```python
from build123d import *

# Parameters (mm, degrees)
BOSS_EXTRUDE1_DEPTH = 1
SKETCH3_R           = 6.8
CUT_EXTRUDE1_DEPTH  = 10


with BuildPart() as part:
    # Sketch1 → Boss-Extrude1 (new body)
    with BuildSketch(Plane(origin=(0, 0, 0), x_dir=(1, 0, 0), z_dir=(0, 1, 0))):
        with BuildLine():
            Line((-58.095782979, 0), (-58.073036978, 0))
            ThreePointArc((-58.073036978, 0), (-57.597480623, -0.18634043), (-57.375111056, -0.646153846))
            ThreePointArc((-57.375111056, -0.646153846), (-48.676683494, -8.393775458), (-40.6, 0))
            Line((-40.6, 0), (-26.532998323, 0))
            ThreePointArc((-26.532998323, 0), (-23.34157463, 1.150998205), (-21.619480115, 4.074074074))
            ThreePointArc((-21.619480115, 4.074074074), (-7.819670385, 20.563383843), (13.44973545, 17.409899952))
            ThreePointArc((13.44973545, 17.409899952), (19.920363156, 17.713546888), (20.660984848, 24.148817192))
            ThreePointArc((20.660984848, 24.148817192), (-17.408618139, 43.353494129), (-53.539393939, 20.711026772))
            ThreePointArc((-53.539393939, 20.711026772), (-54.448939175, 20.409991078), (-54.807009858, 21.298630718))
            ThreePointArc((-54.807009858, 21.298630718), (-6.094732075, 58.483281722), (49.237842792, 32.141481565))
            ThreePointArc((49.237842792, 32.141481565), (49.203069762, 31.327605826), (48.421551499, 31.097753513))
            ThreePointArc((48.421551499, 31.097753513), (38.168934267, 19.364205559), (53.692695632, 20.707760837))
            ThreePointArc((53.692695632, 20.707760837), (54.339746442, 21.20266298), (55.017049011, 20.750043811))
            ThreePointArc((55.017049011, 20.750043811), (57.781950674, 10.894318531), (58.795732172, 0.708433735))
            ThreePointArc((58.795732172, 0.708433735), (58.593730574, 0.208016065), (58.095782979, 0))
            Line((58.095782979, 0), (58.073036978, 0))
            ThreePointArc((58.073036978, 0), (57.597480623, 0.18634043), (57.375111056, 0.646153846))
            ThreePointArc((57.375111056, 0.646153846), (48.676683494, 8.393775458), (40.6, 0))
            Line((40.6, 0), (26.532998323, 0))
            ThreePointArc((26.532998323, 0), (23.34157463, -1.150998205), (21.619480115, -4.074074074))
            ThreePointArc((21.619480115, -4.074074074), (7.819670385, -20.563383843), (-13.44973545, -17.409899952))
            ThreePointArc((-13.44973545, -17.409899952), (-19.920363156, -17.713546888), (-20.660984848, -24.148817192))
            ThreePointArc((-20.660984848, -24.148817192), (17.408618139, -43.353494129), (53.539393939, -20.711026772))
            ThreePointArc((53.539393939, -20.711026772), (54.448939175, -20.409991078), (54.807009858, -21.298630718))
            ThreePointArc((54.807009858, -21.298630718), (6.094732075, -58.483281722), (-49.237842792, -32.141481565))
            ThreePointArc((-49.237842792, -32.141481565), (-49.203069762, -31.327605826), (-48.421551499, -31.097753513))
            ThreePointArc((-48.421551499, -31.097753513), (-38.168934267, -19.364205559), (-53.692695632, -20.707760837))
            ThreePointArc((-53.692695632, -20.707760837), (-54.339746442, -21.20266298), (-55.017049011, -20.750043811))
            ThreePointArc((-55.017049011, -20.750043811), (-57.781950674, -10.894318531), (-58.795732172, -0.708433735))
            ThreePointArc((-58.795732172, -0.708433735), (-58.593730574, -0.208016065), (-58.095782979, 0))
        make_face()
    extrude(amount=BOSS_EXTRUDE1_DEPTH)

    # Sketch3 → Cut-Extrude1 (cut)
    with BuildSketch(Plane(origin=(0, 1, 0), x_dir=(1, 0, 0), z_dir=(0, 1, 0))):
        Circle(SKETCH3_R)
    extrude(amount=-CUT_EXTRUDE1_DEPTH, mode=Mode.SUBTRACT)


solid = part.part
```
Source: CAD feature listing. Evaluate the final solid. Frame: model axes, mm. A direction names the side the tool comes from. Give positions to 0.01 mm unless a question says otherwise; leave off trailing zeros. Loops run counter-clockwise (first coordinate to the right, second up) from the corner with the lowest first, then second, coordinate; pieces in that order, holes last. Notation, with made-up numbers: (9.25, 88.25) - (38.25, 88.25) arc R27 cw to (38.25, 104.25) - close; hole circle Ø6 at (52.5, -11). An arc over 180 degrees is marked (long way). Use CSV: the item, a comma, the result in double quotes.
1) Line query: line 1 (Z direction, x = 0, y = 0.2); line 2 (Z direction, x = -15, y = 0.35); line 3 (X direction, y = 0.7, z = 2.5). Output: solid intervals per line, ascending.
Worked out:
line 1,"z = -58.8 to -40.58, -22 to -6.8, 6.8 to 22, 40.58 to 58.8"
line 2,"z = -56.85 to -43.4, -16.09 to 16.6, 30.97 to 56.85"
line 3,"x = -58.75 to -57.02, -40.98 to -6.32, 6.32 to 22.2"
2) Cut plane D-D (x = 4). Output: boundary loops of the cut face in (y, z), and give its area (3 significant figures).
Worked out:
outline,"(0, -58.66) - (1, -58.66) - (1, -38.82) - (0, -38.82) - close; (0, -21.63) - (1, -21.63) - (1, -5.5) - (0, -5.5) - close; (0, 5.5) - (1, 5.5) - (1, 21.63) - (0, 21.63) - close; (0, 41.88) - (1, 41.88) - (1, 58.66) - (0, 58.66) - close"
area,"68.9 mm^2"
3) Pin query (flat end, axial travel): P1, Ø0.5, axis at x = -34.5, y = 0.5, coming from the -Z side. Return the tip coordinate at first contact, or that it passes through.
Worked out:
P1,"stops at z = -47.8"
4) Cut plane B-B (x = -45). Output: boundary loops of the cut face in (y, z), and give its area (3 significant figures).
Worked out:
outline,"(0, -37.85) - (1, -37.85) - (1, -31.74) - (0, -31.74) - close; (0, 7.39) - (1, 7.39) - (1, 14.79) - (0, 14.79) - close; (0, 31.54) - (1, 31.54) - (1, 37.85) - (0, 37.85) - close"
area,"19.8 mm^2"
5) Mould query, pull axis Z, two halves, no side actions, for faces 1 (the cylindrical face through (-57.755, 0.493, 11.035)), 2 (the cylindrical face through (48.9, 0.5, -8.4)), 3 (the cylindrical face through (8.11, 0.49, 20.45)), 4 (the cylindrical face through (57.755, 0.493, -11.035)). Classes: +Z half, -Z half, draft (parallel to the pull), parting line (faces both ways), or undercut.
Worked out:
face 1,"+Z half"
face 2,"undercut"
face 3,"undercut"
face 4,"-Z half"
6) Set-up query: faces 5 (the flat face through (1, 1, 12)), 6 (the cylindrical face through (23.38, 0.49, 1.12)), 7 (the cylindrical face through (-48.9, 0.5, 8.4)), 8 (the cylindrical face through (-23.38, 0.49, -1.12)). Return all of +Z, -Z, +X, -X, +Y, -Y with unobstructed straight access to the full face (end or side cutting, diameter ignored); none if empty.
Worked out:
face 5,"+Z, -Z, +X, -X, +Y"
face 6,"+X, +Y, -Y"
face 7,"+Y, -Y"
face 8,"-X, +Y, -Y"
7) Cut plane A-A (x = 28). Output: boundary loops of the cut face in (y, z), and give its area (3 significant figures).
Worked out:
outline,"(0, -51.71) - (1, -51.71) - (1, 0) - (0, 0) - close; (0, 41.53) - (1, 41.53) - (1, 51.71) - (0, 51.71) - close"
area,"61.9 mm^2"
